Can you work these out from the model? Positions are in its coordinate system, mm. A direction names the side the tool comes from. Round coordinates to 2 decimals unless told otherwise and drop trailing zeros. Write each loop counter-clockwise with the first axis right and the second up, starting at its lowest first coordinate (ties: lowest second). Pieces come first, ordered by that corner, then holes. Notation, with made-up numbers: M 39.5,81 L 53.5,81 A17 ccw 53.5,106 Z; hole C 8.5,52.5 d2. An arc over 180 degrees is marked long. Answer in a Markdown table with one row per item. Add a question column.
(1) Suppose I cut it at B-B, the plane x = 232.5. Write out the boundary of the cut face in (y, z), then the cut area to 3 significant figures.
(2) If we mould it in two halves opening along Y, with no side actions, what happens to faces 1 (the face through (-275, 3, -1)), 2 (the face through (4, 73, -195)), 3 (the face through (4, 5, 2))? For each: released by +Y, released by -Y, zero draft, split by the parting line, or undercut.
(3) Suppose I cut it at A-A, the plane y = 107.5. Write out the boundary of the cut face in (x, z).
(4) If I drill on probe 1 along Z at (x, y) = (185, 117.9); probe 2 along X at (y, z) = (3.4, 162.5); probe 3 along X at (y, z) = (97, -197.1), over which ranges is the centre line in solid material (lowest first)?
(5) I'm going to push flat-ended pins straight in: pin 1 (4 mm diameter, centred on x = -120, z = 130, fed in from +Y); pin 2 (3.5 mm diameter, centred on x = 65, z = -188, fed in from +Y); pin 3 (15.5 mm diameter, centred on x = 11, z = -190, fed in from -Y) (3 decimals); pin 4 (9.5 mm diameter, centred on x = -65, z = -188, fed in from +Y). Where does each tip first touch, or does it pass through?
(6) Suppose I cut it at C-C, the plane y = 62. Write out the boundary of the cut face in (x, z).
(7) Suppose I cut it at D-D, the plane x = 0. Write out the boundary of the cut face in (y, z).
(8) For faces 4 (the face through (3.85, 8.555, 190.979)), 5 (the face through (-7.553, 78.356, 197.513)), 6 (the face through (3.85, 12.129, -187.482)), which set-ups out of +Z, -Z, +X, -X, +Y, -Y let a thin tool reach every point of the face, with its end or its side?
from build123d import *

# Parameters (mm, degrees)
EXTRUDE_1_DEPTH     = 275
SKETCH_6_R          = 25.5
CUT_EXTRUDE_3_DEPTH = 50
SKETCH_11_R         = 2
SKETCH_11_R_2       = 3
CUT_EXTRUDE_4_DEPTH = 10
SKETCH_12_R         = 3
CUT_EXTRUDE_5_DEPTH = 501.02499951
SKETCH_13_R         = 3
CUT_EXTRUDE_6_DEPTH = 13
SKETCH_14_R         = 3
CUT_EXTRUDE_7_DEPTH = 13


with BuildPart() as part:
    # 草图1 → 凸台-拉伸1 (new, symmetric)
    with BuildSketch(Plane(origin=(0, 0, 0), x_dir=(0, 0, -1), z_dir=(1, 0, 0))):
        with BuildLine():
            Line((0, 0), (-170, 0))
            ThreePointArc((-170, 0), (-191.213203436, 8.786796564), (-200, 30))
            Line((-200, 30), (-200, 120))
            Line((-200, 120), (-181, 120))
            Line((-181, 120), (-181, 117))
            Line((-181, 117), (-195, 117))
            Line((-195, 117), (-195, 115))
            Line((-195, 115), (-195, 30))
            ThreePointArc((-195, 30), (-187.67766953, 12.32233047), (-170, 5))
            Line((-170, 5), (0, 5))
            Line((0, 5), (170, 5))
            ThreePointArc((170, 5), (187.67766953, 12.32233047), (195, 30))
            Line((195, 30), (195, 115))
            Line((195, 115), (195, 117))
            Line((195, 117), (181, 117))
            Line((181, 117), (181, 120))
            Line((181, 120), (200, 120))
            Line((200, 120), (200, 30))
            ThreePointArc((200, 30), (191.213203436, 8.786796564), (170, 0))
            Line((170, 0), (0, 0))
        make_face()
    extrude(amount=EXTRUDE_1_DEPTH, both=True)

    # 草图6 → 切除-拉伸3 (cut)
    with BuildSketch(Plane.XY.offset(200)):
        with Locations(Location((0, 54, 0), (0, 0, 289.749922796))):
            Circle(SKETCH_6_R)
    extrude(amount=-CUT_EXTRUDE_3_DEPTH, mode=Mode.SUBTRACT)

    # 草图11 → 切除-拉伸4 (cut)
    with BuildSketch(Plane.XZ):
        with Locations(Location((-23, 125, 0), (0, 0, 270))):
            Circle(SKETCH_11_R)
        with Locations(Location((-36, 162.5, 0), (0, 0, 270))):
            Circle(SKETCH_11_R_2)
        with Locations(Location((-36, 87.5, 0), (0, 0, 270))):
            Circle(SKETCH_11_R_2)
        with Locations(Location((36, 87.5, 0), (0, 0, 90))):
            Circle(SKETCH_11_R_2)
        with Locations(Location((36, 162.5, 0), (0, 0, 90))):
            Circle(SKETCH_11_R_2)
        with Locations(Location((23, 125, 0), (0, 0, 90))):
            Circle(SKETCH_11_R)
    extrude(amount=-CUT_EXTRUDE_4_DEPTH, mode=Mode.SUBTRACT)

    # 草图12 → 切除-拉伸5 (cut, through all)
    with BuildSketch(Plane(origin=(0, 0, -200), x_dir=(-1, 0, 0), z_dir=(0, 0, -1))):
        with Locations(Location((-265, 97, 0), (0, 0, 90))):
            Circle(SKETCH_12_R)
        with Locations(Location((-265, 76, 0), (0, 0, 90))):
            Circle(SKETCH_12_R)
    cut_extrude_5 = extrude(amount=-CUT_EXTRUDE_5_DEPTH, mode=Mode.SUBTRACT)

    # 镜向1: 切除-拉伸5 across plane
    add(cut_extrude_5.mirror(Plane(origin=(0, 0, 0), x_dir=(0, 0, 1), z_dir=(1, 0, 0))), mode=Mode.SUBTRACT)

    # 草图13 → 切除-拉伸6 (cut)
    with BuildSketch(Plane.XZ):
        with Locations(Location((-265, 120, 0), (0, 0, 270))):
            Circle(SKETCH_13_R)
        with Locations(Location((-265, 60, 0), (0, 0, 270))):
            Circle(SKETCH_13_R)
        with Locations(Location((-265, -120, 0), (0, 0, 270))):
            Circle(SKETCH_13_R)
        with Locations(Location((-265, -60, 0), (0, 0, 270))):
            Circle(SKETCH_13_R)
    cut_extrude_6 = extrude(amount=-CUT_EXTRUDE_6_DEPTH, mode=Mode.SUBTRACT)

    # 镜向2: 切除-拉伸6 across plane
    add(cut_extrude_6.mirror(Plane(origin=(0, 0, 0), x_dir=(0, 0, 1), z_dir=(1, 0, 0))), mode=Mode.SUBTRACT)

    # 草图14 → 切除-拉伸7 (cut)
    with BuildSketch(Plane(origin=(0, 120, 0), x_dir=(1, 0, 0), z_dir=(0, 1, 0))):
        with Locations(Location((-185, -188, 0), (0, 0, 270))):
            Circle(SKETCH_14_R)
        with Locations(Location((-65, -188, 0), (0, 0, 270))):
            Circle(SKETCH_14_R)
        with Locations(Location((65, -188, 0), (0, 0, 270))):
            Circle(SKETCH_14_R)
        with Locations(Location((185, -188, 0), (0, 0, 270))):
            Circle(SKETCH_14_R)
        with Locations(Location((185, 188, 0), (0, 0, 270))):
            Circle(SKETCH_14_R)
        with Locations(Location((65, 188, 0), (0, 0, 270))):
            Circle(SKETCH_14_R)
        with Locations(Location((-65, 188, 0), (0, 0, 270))):
            Circle(SKETCH_14_R)
        with Locations(Location((-185, 188, 0), (0, 0, 270))):
            Circle(SKETCH_14_R)
    extrude(amount=-CUT_EXTRUDE_7_DEPTH, mode=Mode.SUBTRACT)


solid = part.part
Calculated:
| question | item | result |
|---|---|---|
| 1 | outline | M 0,-170 A30 ccw 30,-200 L 120,-200 L 120,-181 L 117,-181 L 117,-195 L 30,-195 A25 cw 5,-170 L 5,170 A25 cw 30,195 L 117,195 L 117,181 L 120,181 L 120,200 L 30,200 A30 ccw 0,170 Z |
| 1 | area | 3,120 mm² |
| 2 | face 1 | zero draft |
| 2 | face 2 | undercut |
| 2 | face 3 | released by +Y |
| 3 | outline | M -275,-200 L 275,-200 L 275,-195 L -275,-195 Z; M -275,195 L 275,195 L 275,200 L -275,200 Z |
| 4 | probe 1 | -200 to -191, -185 to -181, 181 to 185, 191 to 200 |
| 4 | probe 2 | -275 to -39, -33 to 33, 39 to 275 |
| 4 | probe 3 | -275 to -268, -262 to 262, 268 to 275 |
| 5 | pin 1 | y = 5 |
| 5 | pin 2 | y = 14.67 |
| 5 | pin 3 | y = 2.615 |
| 5 | pin 4 | y = 120 |
| 6 | outline | M -275,-200 L 275,-200 L 275,-195 L -275,-195 Z; M -275,195 L -24.21,195 L -24.21,200 L -275,200 Z; M 24.21,195 L 275,195 L 275,200 L 24.21,200 Z |
| 7 | outline | M 0,-170 A30 ccw 30,-200 L 120,-200 L 120,-181 L 117,-181 L 117,-195 L 30,-195 A25 cw 5,-170 L 5,170 A25 cw 28.5,194.95 L 28.5,199.96 A30 ccw 0,170 Z; M 79.5,195 L 117,195 L 117,181 L 120,181 L 120,200 L 79.5,200 Z |
| 8 | face 4 | +Z, +X, -X, -Y |
| 8 | face 5 | +Z |
| 8 | face 6 | +X, -X |
